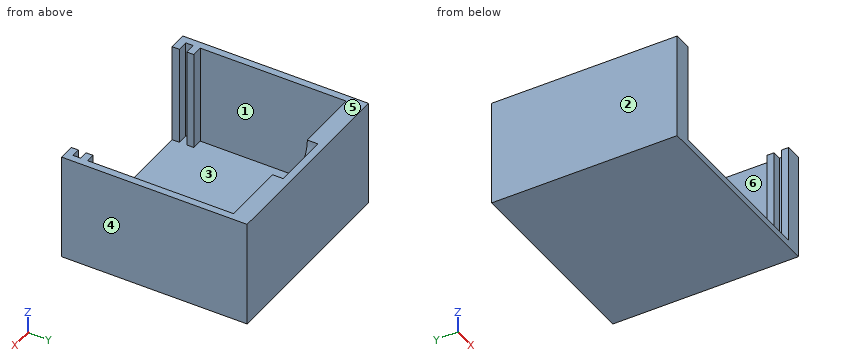
```python
from build123d import *

# Parameters (mm, degrees)
SKETCH1_W           = 56.5
SKETCH1_H           = 60
BOSS_EXTRUDE1_DEPTH = 30
SHELL1_T            = -2
SKETCH2_W           = 52.5
SKETCH2_H           = 3
BOSS_EXTRUDE2_DEPTH = 28
CUT_EXTRUDE5_DEPTH  = 3
SKETCH6_W           = 30
SKETCH6_H           = 2
BOSS_EXTRUDE3_DEPTH = 3
SKETCH7_W           = 30
SKETCH7_H           = 2
BOSS_EXTRUDE4_DEPTH = 3
SKETCH8_W           = 56.5
SKETCH8_H           = 30
CUT_EXTRUDE6_DEPTH  = 7.9


with BuildPart() as part:
    # Sketch1 → Boss-Extrude1 (new body)
    with BuildSketch(Plane.XY):
        with Locations((-28.25, 30)):
            Rectangle(SKETCH1_W, SKETCH1_H)
    extrude(amount=BOSS_EXTRUDE1_DEPTH)

    # Shell1
    shell1_openings = [part.faces().sort_by_distance(p)[0] for p in [
        (-28.25, 30, 30),
    ]]
    offset(amount=SHELL1_T, openings=shell1_openings, kind=Kind.INTERSECTION)

    # Sketch2 → Boss-Extrude2 (add)
    with BuildSketch(Plane.XY.offset(2)):
        with Locations((-28.25, 56.5)):
            Rectangle(SKETCH2_W, SKETCH2_H)
    extrude(amount=BOSS_EXTRUDE2_DEPTH)

    # Sketch3 → Cut-Extrude5 (cut)
    with BuildSketch(Plane.XZ.offset(-55)):
        with BuildLine():
            Line((-36.35, 30), (-20.15, 30))
            ThreePointArc((-20.15, 30), (-28.25, 21.9), (-36.35, 30))
        make_face()
    extrude(amount=-CUT_EXTRUDE5_DEPTH, mode=Mode.SUBTRACT)

    # Sketch6 → Boss-Extrude3 (add)
    with BuildSketch(Plane(origin=(-54.5, 0, 0), x_dir=(0, 0, -1), z_dir=(1, 0, 0))):
        with Locations((-15, 13)):
            Rectangle(SKETCH6_W, SKETCH6_H)
    boss_extrude3 = extrude(amount=BOSS_EXTRUDE3_DEPTH)

    # Sketch7 → Boss-Extrude4 (add)
    with BuildSketch(Plane(origin=(-54.5, 0, 0), x_dir=(0, 0, -1), z_dir=(1, 0, 0))):
        with Locations((-15, 8.9)):
            Rectangle(SKETCH7_W, SKETCH7_H)
    boss_extrude4 = extrude(amount=BOSS_EXTRUDE4_DEPTH)

    # Mirror1: Boss-Extrude3, Boss-Extrude4 across plane
    add(boss_extrude3.mirror(Plane(origin=(-28, 0, 0), x_dir=(0, 0, 1), z_dir=(1, 0, 0))))
    add(boss_extrude4.mirror(Plane(origin=(-28, 0, 0), x_dir=(0, 0, 1), z_dir=(1, 0, 0))))

    # Sketch8 → Cut-Extrude6 (cut)
    with BuildSketch(Plane.XZ):
        with Locations((-28.25, 15)):
            Rectangle(SKETCH8_W, SKETCH8_H)
    extrude(amount=-CUT_EXTRUDE6_DEPTH, mode=Mode.SUBTRACT)


solid = part.part
```
For this review, take the finished solid that the model builds, in its own axes (mm). Face numbers are marked on the shaded views. A direction names the side the tool comes from. Coordinates: 2 decimals unless noted, no trailing zeros. Loops run counter-clockwise (first coordinate to the right, second up) from the corner with the lowest first, then second, coordinate; pieces in that order, holes last. Notation, with made-up numbers: (47.5, 10) -> (77.5, 10) arc R11 cw to (77.5, 22) -> close; hole circle Ø6 at (53, 88). An arc over 180 degrees is marked (long way). Return JSON: item names as keys, results as strings. Group by question number.
(1) Consider section B-B, the plane y = 27.5. Give the boundary of the cut face in (x, z).
(2) Mouldability with a two-part tool opening along X and no side actions: class the marked faces 1, 2, 3 and 4 as pulls with the +X half, pulls with the -X half, needs draft (parallel to the pull), parting line crosses it, or undercut.
(3) For pin 1 Ø1.5 at (x, z) = (-39.5, 26.5) entering from -Y; pin 2 Ø2 at (x, y) = (-22, 47.5) entering from +Z, all flat-tipped, find the tip position at first contact; note any pin that passes through.
(4) To check wall thickness, follow L1, parallel to Y at x = -53, z = 13; L2, parallel to X at y = 51.5, z = 19.5; L3, parallel to Z at x = -9, y = 11. State the ranges of each line that lie inside material, in increasing order.
(5) Consider section C-C, the plane x = -49. Give the boundary of the cut face in (y, z), plus the area to 3 significant figures.
(6) Tool access review of the marked faces 5 and 6: name each direction out of +Z, -Z, +X, -X, +Y, -Y from which nothing blocks a thin tool from reaching the whole face with its end or side.
(7) Consider section A-A, the plane x = -28.25. Give the boundary of the cut face in (y, z), plus the area to 3 significant figures.
Results below:
{
 "1": {"outline": "(-56.5, 0) -> (0, 0) -> (0, 30) -> (-2, 30) -> (-2, 2) -> (-54.5, 2) -> (-54.5, 30) -> (-56.5, 30) -> close"},
 "2": {"face 1": "undercut", "face 2": "pulls with the -X half", "face 3": "undercut", "face 4": "pulls with the +X half"},
 "3": {"pin 1": "stops at y = 55", "pin 2": "stops at z = 2"},
 "4": {"L1": "y = 7.9 to 9.9, 12 to 14, 55 to 60", "L2": "x = -56.5 to -54.5, -2 to 0", "L3": "z = 0 to 2"},
 "5": {"outline": "(7.9, 0) -> (60, 0) -> (60, 30) -> (55, 30) -> (55, 2) -> (7.9, 2) -> close", "area": "244 mm2"},
 "6": {"face 5": "+Z, +X, -X, +Y, -Y", "face 6": "+Z"},
 "7": {"outline": "(7.9, 0) -> (60, 0) -> (60, 30) -> (58, 30) -> (58, 21.9) -> (55, 21.9) -> (55, 2) -> (7.9, 2) -> close", "area": "220 mm2"}
}
